Could you check a few things on this drawing? It's one solid part, dimensions in mm from its lowest x, y, z. Round coordinates to 2 decimals unless told otherwise and drop trailing zeros. Loops run counter-clockwise (first coordinate to the right, second up) from the corner with the lowest first, then second, coordinate; pieces in that order, holes last. Notation, with made-up numbers: (-24.75, 52.25) -> (-15.75, 52.25) arc R14 cw to (-15.75, 61.25) -> close; hole circle Ø2 at (84, -24). An arc over 180 degrees is marked (long way). Use one line per item in the form item = value. Start each with the question number.
Item 1: If we section it at B-B (x = 47): Write out the boundary of the cut face in (y, z), then the cut area to 3 significant figures.
Item 2: If we section it at A-A (z = 21.5): Write out the boundary of the cut face in (x, y) (1 decimal), then the cut area to 3 significant figures.
Item 3: If I drill on L1, parallel to Y at x = 54.5, z = 19.05; L2, parallel to Y at x = 48, z = 20; L3, parallel to Z at x = 56, y = 136.5, over which ranges is the centre line in solid material (lowest first)? Write a range as [from, to].
Item 4: I'm going to push a flat-ended pin straight in: pin 1 Ø16 at (y, z) = (72.932, 19.05) entering from -X. Where does the tip first touch, or does it pass through?
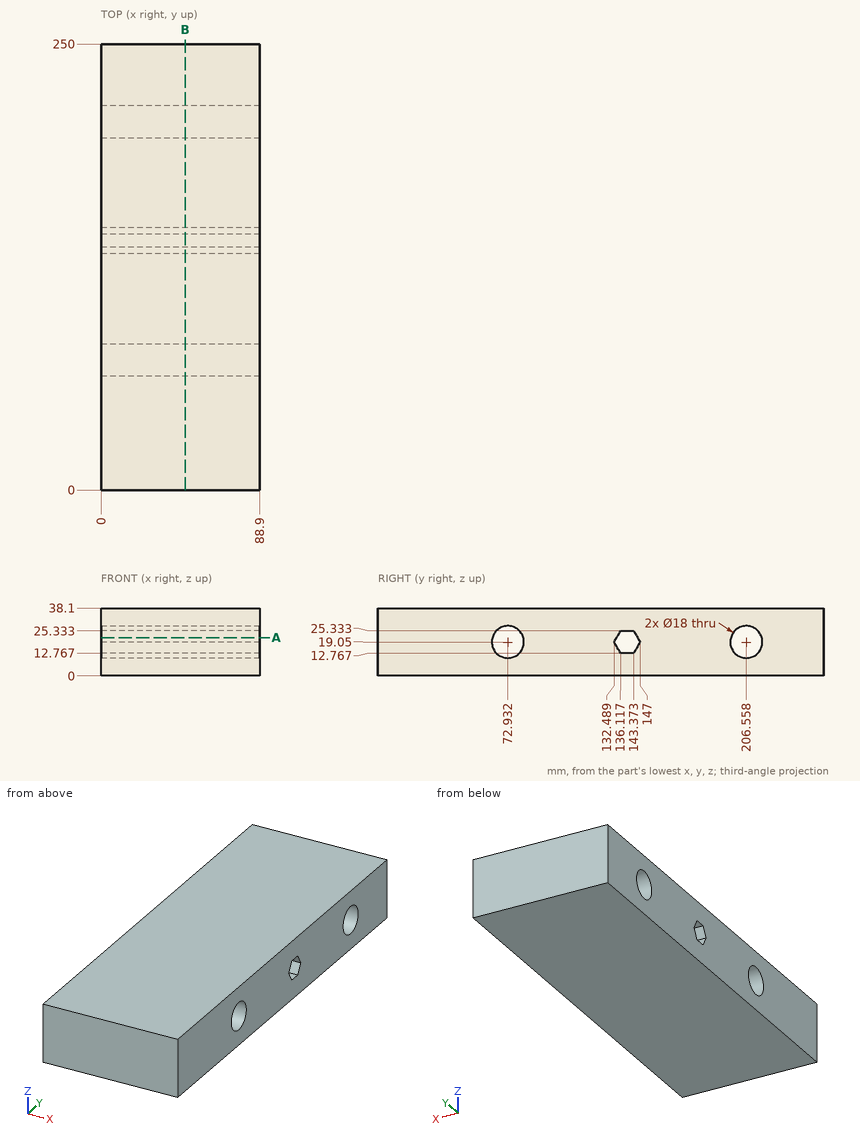
Values found:
q1.outline = (0, 0) -> (250, 0) -> (250, 38.1) -> (0, 38.1) -> close; hole circle Ø18 at (72.93, 19.05); hole (132.49, 19.05) -> (136.12, 12.77) -> (143.37, 12.77) -> (147, 19.05) -> (143.37, 25.33) -> (136.12, 25.33) -> close; hole circle Ø18 at (206.56, 19.05)
q1.area = 8,880 mm2
q2.outline = (0, 0) -> (88.9, 0) -> (88.9, 64.3) -> (0, 64.3) -> close; (0, 81.6) -> (88.9, 81.6) -> (88.9, 133.9) -> (0, 133.9) -> close; (0, 145.6) -> (88.9, 145.6) -> (88.9, 197.9) -> (0, 197.9) -> close; (0, 215.2) -> (88.9, 215.2) -> (88.9, 250) -> (0, 250) -> close
q2.area = 18,100 mm2
q3.L1 = [0, 63.93], [81.93, 132.49], [147, 197.56], [215.56, 250]
q3.L2 = [0, 63.98], [81.88, 133.04], [146.45, 197.61], [215.51, 250]
q3.L3 = [0, 12.77], [25.33, 38.1]
q4.pin_1 = through
